Part model, mm, in its own coordinate system. A direction names the side the tool comes from. Round coordinates to 2 decimals unless told otherwise and drop trailing zeros. Loops run counter-clockwise (first coordinate to the right, second up) from the corner with the lowest first, then second, coordinate; pieces in that order, holes last.
1) Band-saw the part on C-C, the plane x = -30. Write the cut outline in (y, z), then the cut area to 3 significant figures.
2) Probe line 1 (X direction, y = 1, z = 25); line 2 (Y direction, x = 32.75, z = 11); line 3 (X direction, y = 31.5, z = -1). List the from-to ranges inside material, lowest first.
3) Band-saw the part on A-A, the plane z = 25.8. Write the cut outline in (x, y) (3 decimals).
4) Drop flat-ended pins along their axis: P1, Ø1.3, axis at x = 16, y = 8, coming from the -Z side; P2, Ø2, axis at x = 19, z = 5, coming from the -Y side; P3, Ø1.2, axis at x = -14, z = 8.5, coming from the +Y side. Give the stop position or say it passes through.
5) 3-axis set-ups, long thin cutter, end or side, ignore diameter. For faces 1 (the flat face through (-25, 2, 30.3)), 2 (the flat face through (13, 31, 12.7)), 3 (the flat face through (15.58, 16, 15)), 4 (the cylindrical face through (-17.017, 2.194, 5.46)), 5 (the cylindrical face through (22.874, 6.719, 25.701)): which of +Z, -Z, +X, -X, +Y, -Y reach the whole face in a straight line?
6) Mould opens along Z. For faces 6 (the flat face through (0, 35.25, 7)), 7 (the flat face through (-25, 2, 0)), 8 (the flat face through (14, 25.25, 9)) say: +Z half, -Z half, draft (parallel to the pull), parting line (faces both ways), or undercut.
7) Band-saw the part on B-B, the plane x = 2. Write the cut outline in (y, z), then the cut area to 3 significant figures.
from build123d import *

# Parameters (mm, degrees)
SKETCH1_R           = 1.5
BOSS_EXTRUDE1_DEPTH = 30.3
BOSS_EXTRUDE2_DEPTH = 12.15
BOSS_EXTRUDE3_DEPTH = 12.66
FILLET1_R           = 3.875
BOSS_EXTRUDE4_DEPTH = 4.5
SKETCH5_R           = 1.25
CUT_EXTRUDE1_DEPTH  = 10
SKETCH6_R           = 7.75
BOSS_EXTRUDE5_DEPTH = 15.58
FILLET2_R           = 1
FILLET3_R           = 1
SKETCH7_R           = 2
CUT_EXTRUDE2_DEPTH  = 8


with BuildPart() as part:
    # Sketch1 → Boss-Extrude1 (new body)
    with BuildSketch(Plane.XY):
        with BuildLine():
            Line((27.3, -4.5), (32.75, -4.5))
            ThreePointArc((32.75, -4.5), (37.25, 0), (32.75, 4.5))
            Line((32.75, 4.5), (-32.75, 4.5))
            ThreePointArc((-32.75, 4.5), (-37.25, 0), (-32.75, -4.5))
            Line((-32.75, -4.5), (-27.3, -4.5))
            Line((-27.3, -4.5), (-27.3, -1.75))
            Line((-27.3, -1.75), (27.3, -1.75))
            Line((27.3, -1.75), (27.3, -4.5))
        make_face()
        with Locations(Location((-32.75, 0, 0), (0, 0, 180))):
            Circle(SKETCH1_R, mode=Mode.SUBTRACT)
        with Locations(Location((32.75, 0, 0), (0, 0, 180))):
            Circle(SKETCH1_R, mode=Mode.SUBTRACT)
    extrude(amount=BOSS_EXTRUDE1_DEPTH)

    # Sketch2 → Boss-Extrude2 (add, symmetric)
    with BuildSketch(Plane(origin=(0, 0, 0), x_dir=(0, 0, -1), z_dir=(1, 0, 0))):
        with BuildLine():
            Line((-35.05, -1.75), (3.45, -1.75))
            Line((3.45, -1.75), (3.45, 32.25))
            ThreePointArc((3.45, 32.25), (2.571320344, 34.371320344), (0.45, 35.25))
            Line((0.45, 35.25), (-15.05, 35.25))
            ThreePointArc((-15.05, 35.25), (-29.192135624, 29.392135624), (-35.05, 15.25))
            Line((-35.05, 15.25), (-35.05, -1.75))
        make_face()
    extrude(amount=BOSS_EXTRUDE2_DEPTH, both=True)

    # Sketch3 → Boss-Extrude3 (add)
    with BuildSketch(Plane(origin=(0, 35.25, 0), x_dir=(1, 0, 0), z_dir=(0, 1, 0))):
        with BuildLine():
            Line((14, -12.7), (-14, -12.7))
            ThreePointArc((-14, -12.7), (-17.875, -8.825), (-14, -4.95))
            Line((-14, -4.95), (14, -4.95))
            ThreePointArc((14, -4.95), (17.875, -8.825), (14, -12.7))
        make_face()
    extrude(amount=-BOSS_EXTRUDE3_DEPTH)

    # Fillet1
    fillet1_edges = [part.edges().sort_by_distance(p)[0] for p in [
        (-13.075, 22.59, 4.95),
        (-13.075, 22.59, 12.7),
        (13.075, 22.59, 12.7),
        (13.075, 22.59, 4.95),
        (-17.875, 22.59, 8.825),
        (17.875, 22.59, 8.825),
    ]]
    fillet(fillet1_edges, radius=FILLET1_R - 0.0001)  # a hair under: the kernel refuses the full size

    # Sketch4 → Boss-Extrude4 (add)
    with BuildSketch(Plane(origin=(0, 4.5, 0), x_dir=(1, 0, 0), z_dir=(0, 1, 0))):
        with BuildLine():
            Line((-18.375, 0), (18.375, 0))
            ThreePointArc((18.375, 0), (22.875, -4.5), (18.375, -9))
            Line((18.375, -9), (-18.375, -9))
            ThreePointArc((-18.375, -9), (-22.875, -4.5), (-18.375, 0))
        make_face()
        with BuildLine():
            Line((18.375, -30.3), (-18.375, -30.3))
            ThreePointArc((-18.375, -30.3), (-22.875, -25.8), (-18.375, -21.3))
            Line((-18.375, -21.3), (18.375, -21.3))
            ThreePointArc((18.375, -21.3), (22.875, -25.8), (18.375, -30.3))
        make_face()
    extrude(amount=BOSS_EXTRUDE4_DEPTH)

    # Sketch5 → Cut-Extrude1 (cut)
    with BuildSketch(Plane(origin=(0, 35.25, 0), x_dir=(1, 0, 0), z_dir=(0, 1, 0))):
        with Locations(Location((14, -8.825, 0), (0, 0, 270))):
            Circle(SKETCH5_R)
        with Locations(Location((-14, -8.825, 0), (0, 0, 270))):
            Circle(SKETCH5_R)
    extrude(amount=-CUT_EXTRUDE1_DEPTH, mode=Mode.SUBTRACT)

    # Sketch6 → Boss-Extrude5 (add, symmetric)
    with BuildSketch(Plane(origin=(0, 0, 0), x_dir=(0, 0, -1), z_dir=(1, 0, 0))):
        with Locations((-15.15, 15.75)):
            Circle(SKETCH6_R)
    extrude(amount=BOSS_EXTRUDE5_DEPTH, both=True)

    # Fillet2
    fillet2_edges = [part.edges().sort_by_distance(p)[0] for p in [
        (-15.58, 15.75, 22.9),
        (15.58, 15.75, 22.9),
    ]]
    fillet(fillet2_edges, radius=FILLET2_R)

    # Fillet3
    fillet3_edges = [part.edges().sort_by_distance(p)[0] for p in [
        (-12.15, 15.25, -3.45),
        (-12.15, 34.371320344, -2.571320344),
        (-12.15, 35.25, 2.25),
        (12.15, 15.25, -3.45),
        (12.15, 34.371320344, -2.571320344),
        (12.15, 35.25, 2.25),
    ]]
    fillet(fillet3_edges, radius=FILLET3_R)

    # Sketch7 → Cut-Extrude2 (cut)
    with BuildSketch(Plane.XZ.offset(1.75)):
        with Locations(Location((-19, 5.2, 0), (0, 0, 270))):
            Circle(SKETCH7_R)
        with Locations(Location((-19, 25.2, 0), (0, 0, 270))):
            Circle(SKETCH7_R)
        with Locations(Location((19, 5.2, 0), (0, 0, 90))):
            Circle(SKETCH7_R)
        with Locations(Location((19, 25.2, 0), (0, 0, 90))):
            Circle(SKETCH7_R)
    extrude(amount=-CUT_EXTRUDE2_DEPTH, mode=Mode.SUBTRACT)


solid = part.part
Reported:
1. outline: (-4.5, 0) - (4.5, 0) - (4.5, 30.3) - (-4.5, 30.3) - close
1. area: 273 mm2
2. line 1: x = -37.14 to -33.87, -31.63 to -20.99, -17.01 to 17.01, 20.99 to 31.63, 33.87 to 37.14
2. line 2: y = -4.5 to -1.5, 1.5 to 4.5
2. line 3: x = -12.15 to 12.15
3. outline: (-32.75, -4.5) - (-27.3, -4.5) - (-27.3, -1.75) - (-20.908, -1.75) - (-20.908, 6.25) - (-17.092, 6.25) - (-17.092, -1.75) - (17.092, -1.75) - (17.092, 6.25) - (20.908, 6.25) - (20.908, -1.75) - (27.3, -1.75) - (27.3, -4.5) - (32.75, -4.5) arc R4.5 ccw to (32.75, 4.5) - (22.875, 4.5) - (22.875, 9) - (12.15, 9) - (12.15, 32.115) - (-12.15, 32.115) - (-12.15, 9) - (-22.875, 9) - (-22.875, 4.5) - (-32.75, 4.5) arc R4.5 ccw to start; hole circle Ø3 at (-32.75, 0); hole circle Ø3 at (32.75, 0)
4. P1: stops at z = 0
4. P2: stops at y = 6.25
4. P3: stops at y = 25.25
5. face 1: +Z, -X, +Y, -Y
5. face 2: +Z, +X, +Y
5. face 3: +Z, -Z, +X
5. face 4: -Y
5. face 5: +X, +Y
6. face 6: draft
6. face 7: -Z half
6. face 8: undercut
7. outline: (-1.75, -3.45) - (32.25, -3.45) arc R3 ccw to (35.25, -0.45) - (35.25, 15.05) arc R20 ccw to (15.25, 35.05) - (-1.75, 35.05) - close
7. area: 1,340 mm2
